Autodesk Fusion 360 part; units mm, degrees
sketch "3D-printed conduit top outline" plane through (0, 0, 0) normal (0, 1, 0) x (1, 0, 0)
  line L0 (0, 0) -> (16, 0)
  line L1 (16, 0) -> (16, -2)
  line L2 (16, -2) -> (0, -2)
  line L3 (0, -2) -> (0, 0)
  dimension "d7" = 16
  dimension "d8" = 2
extrude "Extrude1" add sketch "3D-printed conduit top outline" along normal blind 161.69
sketch "Magnet holes" plane through (0, 0, 2) normal (0, 0, 1) x (-1, 0, 0)
  line L0 (0, 0) -> (-16, 0)
  line L1 (-16, 0) -> (-16, -161.69)
  line L2 (-16, -161.69) -> (0, -161.69)
  line L3 (0, -161.69) -> (0, 0)
  circle A0 centre (-2.5, -2.5) radius 2.5
  circle A1 centre (-13.5, -2.5) radius 2.5
  circle A2 centre (-2.5, -2.5) radius 1.75
  circle A3 centre (-13.5, -2.5) radius 1.75
  circle A4 centre (-2.5, -54.73) radius 1.75
  circle A5 centre (-2.5, -54.73) radius 2.5
  circle A6 centre (-13.5, -54.73) radius 2.5
  circle A7 centre (-13.5, -54.73) radius 1.75
  circle A8 centre (-2.5, -106.96) radius 1.75
  circle A9 centre (-2.5, -106.96) radius 2.5
  circle A10 centre (-13.5, -106.96) radius 2.5
  circle A11 centre (-13.5, -106.96) radius 1.75
  circle A12 centre (-2.5, -159.19) radius 1.75
  circle A13 centre (-2.5, -159.19) radius 2.5
  circle A14 centre (-13.5, -159.19) radius 2.5
  circle A15 centre (-13.5, -159.19) radius 1.75
  dimension "d11" = 5
  dimension "d12" = 5
  dimension "d13" = 3.5
  dimension "d14" = 3.5
  dimension "d17" = 0
  dimension "d18" = -156.69
extrude "Extrude2" cut sketch "Magnet holes" against normal blind 1 contours A2 | A3 | A4 | A7 | A8 | A11 | A12 | A15
sketch "Support rib" plane through (0, 0, 2) normal (0, 0, 1) x (-1, 0, 0)
  line L0 (0, 0) -> (-16, 0)
  line L1 (-16, 0) -> (-16, -161.69)
  line L2 (-16, -161.69) -> (0, -161.69)
  line L3 (0, -161.69) -> (0, 0)
  circle A0 centre (-13.5, -159.19) radius 1.75
  circle A1 centre (-13.5, -54.73) radius 1.75
  circle A2 centre (-2.5, -2.5) radius 1.75
  circle A3 centre (-2.5, -106.96) radius 1.75
  circle A4 centre (-2.5, -159.19) radius 1.75
  circle A5 centre (-2.5, -54.73) radius 1.75
  circle A6 centre (-13.5, -2.5) radius 1.75
  circle A7 centre (-13.5, -106.96) radius 1.75
  line L4 (-5.5, 0) -> (-10.5, 0)
  line L5 (-10.5, 0) -> (-10.5, -161.69)
  line L6 (-10.5, -161.69) -> (-5.5, -161.69)
  line L7 (-5.5, -161.69) -> (-5.5, 0)
  dimension "d23" = 5
  dimension "d24" = 5.5
  dimension "d25" = 5.5
extrude "Extrude3" add sketch "Support rib" along normal blind 3 contours L0 L2 L4 L5 L6 L7
chamfer "Chamfer1" distance 0.5 angle 45 2 edges at (5.5, 80.845, 5) (10.5, 80.845, 5)
equation "conduit_length = 161.69 mm"
equation "conduit_width = 16 mm"
equation "conduit_wall_thickness = 2 mm"
equation "magnet_diameter = 3 mm"
equation "magnet_height = 1 mm"
equation "d7 = conduit_width"
equation "d8 = conduit_wall_thickness"
equation "d9 = conduit_length"
equation "d11 = magnet_diameter + 2 mm"
equation "d12 = magnet_diameter + 2 mm"
equation "d13 = magnet_diameter + 0.5 mm"
equation "d14 = magnet_diameter + 0.5 mm"
equation "d18 = -conduit_length + magnet_diameter + 2 mm"
equation "rib_width = 5 mm"
equation "rib_height = 3 mm"
equation "d23 = rib_width"
equation "d24 = ( conduit_width - rib_width ) / 2"
equation "d26 = rib_height"
equation "rib_chamfer = 0.5 mm"
equation "d29 = rib_chamfer"
For this review, take the finished solid that the model builds, in its own axes (mm). A direction names the side the tool comes from. Round coordinates to 2 decimals unless told otherwise and drop trailing zeros. Loops run counter-clockwise (first coordinate to the right, second up) from the corner with the lowest first, then second, coordinate; pieces in that order, holes last. Notation, with made-up numbers: (32.5, 79.5) - (50.5, 79.5) arc R21 ccw to (50.5, 102.5) - close; hole circle Ø6 at (-30, -9.75). An arc over 180 degrees is marked (long way). Put each result on its own line as item: value. Start each with the question number.
1. For probe 1 along X at (y, z) = (159.19, 1.4); probe 2 along Y at (x, z) = (2.5, 1.8); probe 3 along X at (y, z) = (58, 3.4), list the stretches that pass through material, from the lowest coordinate up. Write a range as [from, to].
2. Consider section B-B on y = 54.73. State the section outline as (x, z) points.
3. Consider section A-A on x = 13.5. State the section outline as (y, z) points, plus the area to 3 significant figures.
4. Mouldability with a two-part tool opening along X and no side actions: class faces 4 (the flat face through (3, 107, 1)), 5 (the flat face through (5.5, 82, 3)), 6 (the flat face through (13, 80, 2)) as +X half, -X half, draft (parallel to the pull), parting line (faces both ways), or undercut.
5. Consider section C-C on z = 3.7. State the section outline as (x, y) points, plus the area to 3 significant figures.
6. For faces 1 (the flat face through (8, 161.69, 2)), 2 (the flat face through (3, 2, 1)), 3 (the flat face through (3, 80, 2)), list the 3-axis set-ups (+Z, -Z, +X, -X, +Y, -Y) from which the entire face can be reached by the end or side of a thin tool; tool diameter is ignored.
7. Insertion check: P1, Ø3, axis at x = 13.5, y = 54.73, coming from the -Z side; P2, Ø1, axis at x = 3, y = 3, coming from the +Z side; P3, Ø4.5, axis at x = 2.5, y = 54.73, coming from the +Z side. Each pin has a flat end and moves straight along its axis. Give the tip position at first contact, or say it passes through.
Result sheet:
1. probe 1: [0, 0.75], [4.25, 11.75], [15.25, 16]
1. probe 2: [0, 0.75], [4.25, 52.98], [56.48, 105.21], [108.71, 157.44], [160.94, 161.69]
1. probe 3: [5.5, 10.5]
2. outline: (0, 0) - (16, 0) - (16, 2) - (15.25, 2) - (15.25, 1) - (11.75, 1) - (11.75, 2) - (10.5, 2) - (10.5, 4.5) - (10, 5) - (6, 5) - (5.5, 4.5) - (5.5, 2) - (4.25, 2) - (4.25, 1) - (0.75, 1) - (0.75, 2) - (0, 2) - close
3. outline: (0, 0) - (161.69, 0) - (161.69, 2) - (160.94, 2) - (160.94, 1) - (157.44, 1) - (157.44, 2) - (108.71, 2) - (108.71, 1) - (105.21, 1) - (105.21, 2) - (56.48, 2) - (56.48, 1) - (52.98, 1) - (52.98, 2) - (4.25, 2) - (4.25, 1) - (0.75, 1) - (0.75, 2) - (0, 2) - close
3. area: 309 mm^2
4. face 4: undercut
4. face 5: -X half
4. face 6: draft
5. outline: (5.5, 0) - (10.5, 0) - (10.5, 161.69) - (5.5, 161.69) - close
5. area: 808 mm^2
6. face 1: +Z, -Z, +X, -X, +Y
6. face 2: +Z
6. face 3: +Z, -X, +Y, -Y
7. P1: z = 0
7. P2: z = 1
7. P3: z = 2
